Source: three-view drawing plus pictorial views. Frame: mm from the lowest corner of the part. A direction names the side the tool comes from. Round coordinates to 2 decimals unless told otherwise and drop trailing zeros. Loops run counter-clockwise (first coordinate to the right, second up) from the corner with the lowest first, then second, coordinate; pieces in that order, holes last. Notation, with made-up numbers: M -7.75,62 L 5.25,62 A21 ccw 5.25,99 Z; hole C -10,14.25 d11. An arc over 180 degrees is marked long. Write each question's results on one line, items separated by ' | '.
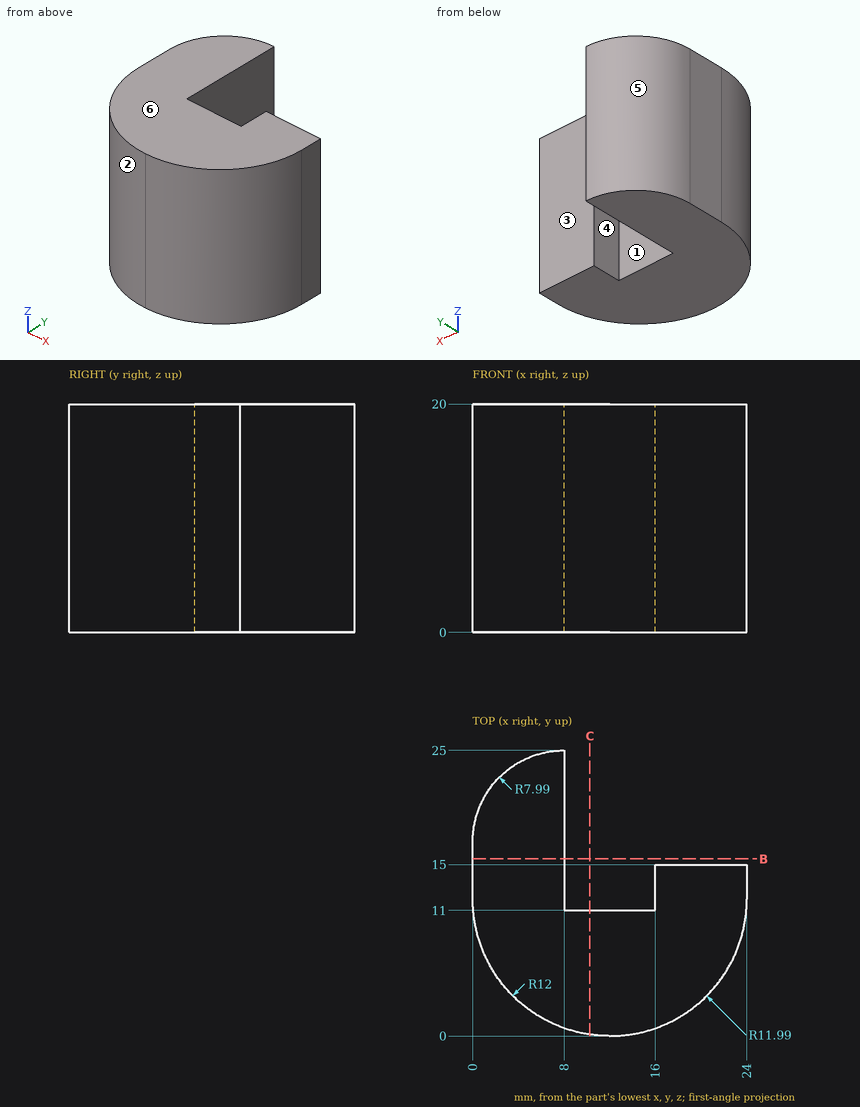
1. Pin query (flat end, axial travel): P1, Ø2.5, axis at x = 14, z = 7.5, coming from the +Y side; P2, Ø8, axis at x = 14.5, z = 10.5, coming from the +Y side. Return the tip coordinate at first contact, or that it passes through.
Answer key:
P1: stops at y = 11 | P2: stops at y = 15
2. Section C-C (x = 10.25). Output: boundary loops of the cut face in (y, z), then the cut area to 3 significant figures.
Answer key:
outline: M 0.13,0 L 11,0 L 11,20 L 0.13,20 Z | area: 217 mm²
3. Ray query, probe 1 along X at (y, z) = (13.5, 3); probe 2 along X at (y, z) = (15.5, 10); probe 3 along Y at (x, z) = (3.5, 1). Return the intervals inside material, ascending.
Answer key:
probe 1: x = 0 to 8, 16 to 24 | probe 2: x = 0 to 8 | probe 3: y = 3.53 to 23.62
4. Access query for the marked faces 1, 2 and 3. Directions: +Z, -Z, +X, -X, +Y, -Y. A direction counts if a zero-diameter tool reaches every point of the face in a straight line with its end or side. Return the directions, or none.
Answer key:
face 1: +Z, -Z, +Y | face 2: +Z, -Z, -X, -Y | face 3: +Z, -Z, +X, +Y
5. Section B-B (y = 15.5). Output: boundary loops of the cut face in (x, z).
Answer key:
outline: M 0,0 L 8,0 L 8,20 L 0,20 Z
6. Draft query along X for the marked faces 4, 5 and 6. Return one class per face: pulls with the +X half, pulls with the -X half, needs draft (parallel to the pull), parting line crosses it, or undercut.
Answer key:
face 4: undercut | face 5: pulls with the -X half | face 6: needs draft
